For this review, use the dimensioned drawing (mm, ordinates from the lowest corner) and the shaded views. A direction names the side the tool comes from. Give positions to 0.01 mm unless a question says otherwise; leave off trailing zeros. Order: outer loops, then holes, each group sorted by start corner. A loop starts at its lowest first (then second) coordinate and runs counter-clockwise, first axis right, second up. Notation, with made-up numbers: (53.5, 9) - (81.5, 9) arc R21 ccw to (81.5, 43) - close; hole circle Ø1 at (-35.75, 10). An arc over 180 degrees is marked (long way). Use a Markdown table: item, result. Add a question column.
1) We need section C-C on z = 25. Write out the cut boundary in (x, y).
2) We need section B-B on y = 25. Write out the cut boundary in (x, z), then the cut area to 3 significant figures.
3) We need section D-D on y = 146. Write out the cut boundary in (x, z), then the cut area to 3 significant figures.
4) Clearance check with flat-ended pins moving along their axes: P1, Ø2, axis at x = 24.5, y = 32.5, coming from the -Z side; P2, Ø1, axis at y = 84, z = 19.5, coming from the +X side; P3, Ø6.5, axis at y = 135, z = 25, coming from the -X side; P4, Ø4, axis at x = 25, y = 135, coming from the +Z side. State where each tip first meets the part, or that it passes through.
5) We need section A-A on x = 25. Write out the cut boundary in (y, z).
6) Machinability: for the marked faces 1 and 2, which of the approach directions +Z, -Z, +X, -X, +Y, -Y give a long, thin tool a straight path to every point of the face, cutting with its end or side? Answer none if there is none.
7) Wall thickness on L1, parallel to Y at x = 25, z = 46.95; L2, parallel to X at y = 135, z = 48: over which ranges is each line inside the solid? List them lowest first.
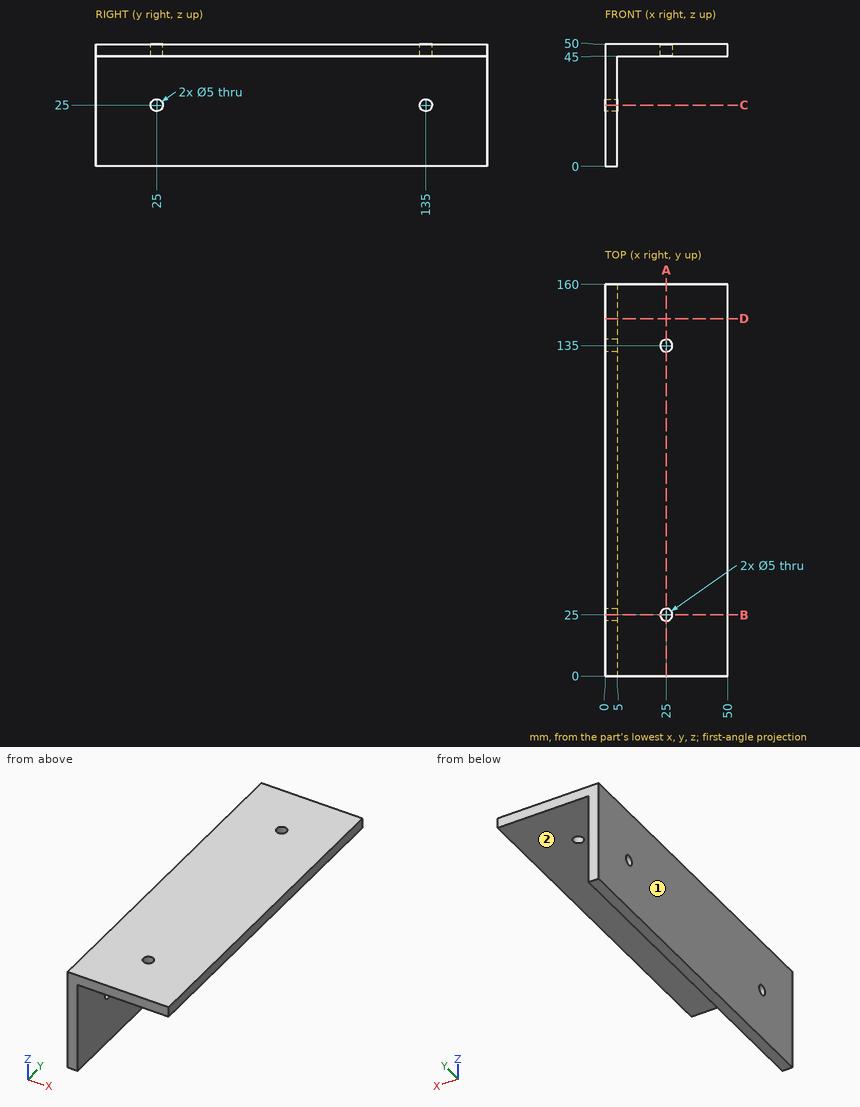
Checked values:
| question | item | result |
|---|---|---|
| 1 | outline | (0, 0) - (5, 0) - (5, 22.5) - (0, 22.5) - close; (0, 27.5) - (5, 27.5) - (5, 132.5) - (0, 132.5) - close; (0, 137.5) - (5, 137.5) - (5, 160) - (0, 160) - close |
| 2 | outline | (0, 0) - (5, 0) - (5, 22.5) - (0, 22.5) - close; (0, 27.5) - (5, 27.5) - (5, 45) - (22.5, 45) - (22.5, 50) - (0, 50) - close; (27.5, 45) - (50, 45) - (50, 50) - (27.5, 50) - close |
| 2 | area | 425 mm² |
| 3 | outline | (0, 0) - (5, 0) - (5, 45) - (50, 45) - (50, 50) - (0, 50) - close |
| 3 | area | 475 mm² |
| 4 | P1 | z = 45 |
| 4 | P2 | x = 5 |
| 4 | P3 | x = 0 |
| 4 | P4 | through |
| 5 | outline | (0, 45) - (22.5, 45) - (22.5, 50) - (0, 50) - close; (27.5, 45) - (132.5, 45) - (132.5, 50) - (27.5, 50) - close; (137.5, 45) - (160, 45) - (160, 50) - (137.5, 50) - close |
| 6 | face 1 | +Z, -Z, -X, +Y, -Y |
| 6 | face 2 | -Z, +X, +Y, -Y |
| 7 | L1 | 0 to 22.5, 27.5 to 132.5, 137.5 to 160 |
| 7 | L2 | 0 to 22.5, 27.5 to 50 |
